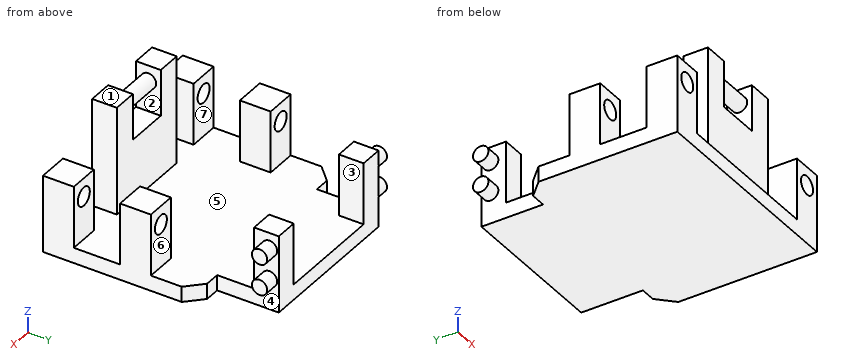
from build123d import *

# Parameters (mm, degrees)
F0_W      = 50
F0_H      = 20
F1_DEPTH  = 8
F2_R      = 2.5
F3_DEPTH  = 5
F4_R      = 2.5
F5_DEPTH  = 5
F6_W      = 35
F6_H      = 30
F7_DEPTH  = 25
F9_DEPTH  = 5
F10_W     = 8
F10_H     = 8
F11_DEPTH = 35
F12_R     = 2.5
F13_DEPTH = 14
F14_W     = 10
F14_H     = 10
F15_DEPTH = 20
F16_R     = 3
F17_DEPTH = 50
F18_SIZE  = 5
F19_SIZE  = 5
F20_W     = 14
F20_H     = 8
F21_DEPTH = 20


with BuildPart() as f1:
    # F0 (on Front) → F1 (new body)
    with BuildSketch(Plane.XZ):
        Rectangle(F0_W, F0_H)
    extrude(amount=F1_DEPTH)

    # F2 (on face) → F3 (join)
    with BuildSketch(Plane(origin=(-25, 0, 0), x_dir=(0, -1, 0), z_dir=(-1, 0, 0))):
        with Locations((3, 5)):
            Circle(F2_R)
        with Locations((3, -5)):
            Circle(F2_R)
    extrude(amount=F3_DEPTH)

    # F4 (on face) → F5 (join)
    with BuildSketch(Plane.YZ.offset(25)):
        with Locations((-3, 5)):
            Circle(F4_R)
        with Locations((-3, -5)):
            Circle(F4_R)
    extrude(amount=F5_DEPTH)

    # F6 (on face) → F7 (cut)
    with BuildSketch(Plane.XZ.offset(8)):
        with Locations((0, 5)):
            Rectangle(F6_W, F6_H)
    extrude(amount=-F7_DEPTH, mode=Mode.SUBTRACT)

    # F8 (on face) → F9 (join)
    with BuildSketch(Plane(origin=(0, 0, -10), x_dir=(1, 0, 0), z_dir=(0, 0, -1))):
        Polygon((-25, 20), (-25, 0), (25, 0), (25, 20), (35, 20), (35, 70), (-35, 70), (-35, 20), align=None)
    extrude(amount=F9_DEPTH)

    # F10 (on face) → F11 (join)
    with BuildSketch(Plane.XY.offset(-10)):
        with Locations((-11, -63)):
            Rectangle(F10_W, F10_H)
        with Locations((11, -63)):
            Rectangle(F10_W, F10_H)
    extrude(amount=F11_DEPTH)

    # F12 (on face) → F13 (join, through all)
    with BuildSketch(Plane(origin=(7, 0, 0), x_dir=(0, -1, 0), z_dir=(-1, 0, 0))):
        with Locations((63, 20)):
            Circle(F12_R)
    extrude(amount=F13_DEPTH)

    # F14 (on face) → F15 (join)
    with BuildSketch(Plane.XY.offset(-10)):
        with Locations((-30, -65)):
            Rectangle(F14_W, F14_H)
        with Locations((30, -65)):
            Rectangle(F14_W, F14_H)
        with Locations((30, -40)):
            Rectangle(F14_W, F14_H)
        with Locations((-30, -40)):
            Rectangle(F14_W, F14_H)
    extrude(amount=F15_DEPTH)

    # F16 (on face) → F17 (cut)
    with BuildSketch(Plane.XZ.offset(70)):
        with Locations((30, 4)):
            Circle(F16_R)
        with Locations((-30, 4)):
            Circle(F16_R)
    extrude(amount=-F17_DEPTH, mode=Mode.SUBTRACT)

    # F18
    f18_edges = [f1.edges().sort_by_distance(p)[0] for p in [
        (-35, -20, -12.5),
    ]]
    chamfer(f18_edges, length=F18_SIZE)

    # F19
    f19_edges = [f1.edges().sort_by_distance(p)[0] for p in [
        (35, -20, -12.5),
    ]]
    chamfer(f19_edges, length=F19_SIZE)

    # F20 (on face) → F21 (join)
    with BuildSketch(Plane.XY.offset(-10)):
        with Locations((0, -63)):
            Rectangle(F20_W, F20_H)
    extrude(amount=F21_DEPTH)


solid = f1.part
Build history of the part. All positions in model axes, mm. Face numbers are marked on the shaded views. A direction names the side the tool comes from. Give positions to 0.01 mm unless a question says otherwise; leave off trailing zeros. Order: outer loops, then holes, each group sorted by start corner. A loop starts at its lowest first (then second) coordinate and runs counter-clockwise, first axis right, second up. Notation, with made-up numbers: M -4.75,1.5 L 51.25,1.5 A18 ccw 51.25,21.5 Z; hole C 59.5,-20 d9. An arc over 180 degrees is marked long. Use one line per item in the form item = value.
Q1. Slice it at A-A, the plane z = -1. Write the cut outline in (x, y), and give its area (3 significant figures).
Conclusion:
outline = M -35,-70 L -25,-70 L -25,-60 L -35,-60 Z; M -35,-45 L -25,-45 L -25,-35 L -35,-35 Z; M -25,-8 L -17.5,-8 L -17.5,0 L -25,0 Z; M -15,-67 L 15,-67 L 15,-59 L -15,-59 Z; M 17.5,-8 L 25,-8 L 25,0 L 17.5,0 Z; M 25,-70 L 35,-70 L 35,-60 L 25,-60 Z; M 25,-45 L 35,-45 L 35,-35 L 25,-35 Z
area = 760 mm2
Q2. Slice it at D-D, the plane y = -3. Write the cut outline in (x, z), and give its area (3 significant figures).
Conclusion:
outline = M -30,-7.5 L -25,-7.5 L -25,-15 L 25,-15 L 25,-7.5 L 30,-7.5 L 30,-2.5 L 25,-2.5 L 25,2.5 L 30,2.5 L 30,7.5 L 25,7.5 L 25,10 L 17.5,10 L 17.5,-10 L -17.5,-10 L -17.5,10 L -25,10 L -25,7.5 L -30,7.5 L -30,2.5 L -25,2.5 L -25,-2.5 L -30,-2.5 Z
area = 650 mm2
Q3. Wall check: probe 1 along X at (y, z) = (-5.5, -6.5); probe 2 along Z at (x, y) = (30, -67.75); probe 3 along X at (y, z) = (-61, 4.5). Give the ranges that are in metal, low to high.
Conclusion:
probe_1 = -25 to -17.5, 17.5 to 25
probe_2 = -15 to 1, 7 to 10
probe_3 = -35 to -32.96, -27.04 to -25, -15 to 15, 25 to 27.04, 32.96 to 35
Q4. Slice it at C-C, the plane x = -28. Write the cut outline in (y, z).
Conclusion:
outline = M -70,-15 L -20,-15 L -20,-10 L -35,-10 L -35,1.76 L -45,1.76 L -45,-10 L -60,-10 L -60,1.76 L -70,1.76 Z; M -70,6.24 L -60,6.24 L -60,10 L -70,10 Z; M -45,6.24 L -35,6.24 L -35,10 L -45,10 Z; C -3,-5 d5; C -3,5 d5
Q5. Pull direction Z, two halves, no side cores. Call the marked faces 1, 2 and 3: released by +Z, released by -Z, zero draft, split by the parting line, or undercut.
Conclusion:
face_1 = released by +Z
face_2 = undercut
face_3 = zero draft
Q6. Slice it at B-B, the plane z = 12.5. Write the cut outline in (x, y), and give its area (3 significant figures).
Conclusion:
outline = M -15,-67 L -7,-67 L -7,-59 L -15,-59 Z; M 7,-67 L 15,-67 L 15,-59 L 7,-59 Z
area = 128 mm2
Q7. Which spindle directions (+Z, -Z, +X, -X, +Y, -Y) get a long thin tool onto all of the face, cutting with end or side? Do the marked faces 4, 5, 6 and 7. Say none if no direction does.
Conclusion:
face_4 = +X
face_5 = +Z
face_6 = +Z, +X, -X
face_7 = +Z, -X
Q8. Pin check, flat tips, straight feed: P1, Ø6, axis at x = -15, z = 7, coming from the -Y side; P2, Ø3, axis at x = -28.5, y = -65, coming from the +Z side; P3, Ø6.5, axis at y = -64.5, z = 17, coming from the -X side. Stop position of each tip, or through.
Conclusion:
P1 = -67
P2 = 10
P3 = -15
